Geometry: see drawing. Coordinates: mm, zero at the bounding-box minimum. A direction names the side the tool comes from. Give positions to 0.01 mm unless a question says otherwise; leave off trailing zeros. Loops run counter-clockwise (first coordinate to the right, second up) from the corner with the lowest first, then second, coordinate; pieces in that order, holes last. Notation, with made-up numbers: M 89,17 L 98,17 A22 ccw 98,54 Z; hole C -4.5,6 d2. An arc over 180 degrees is marked long. Put each result on its own line as item: value.
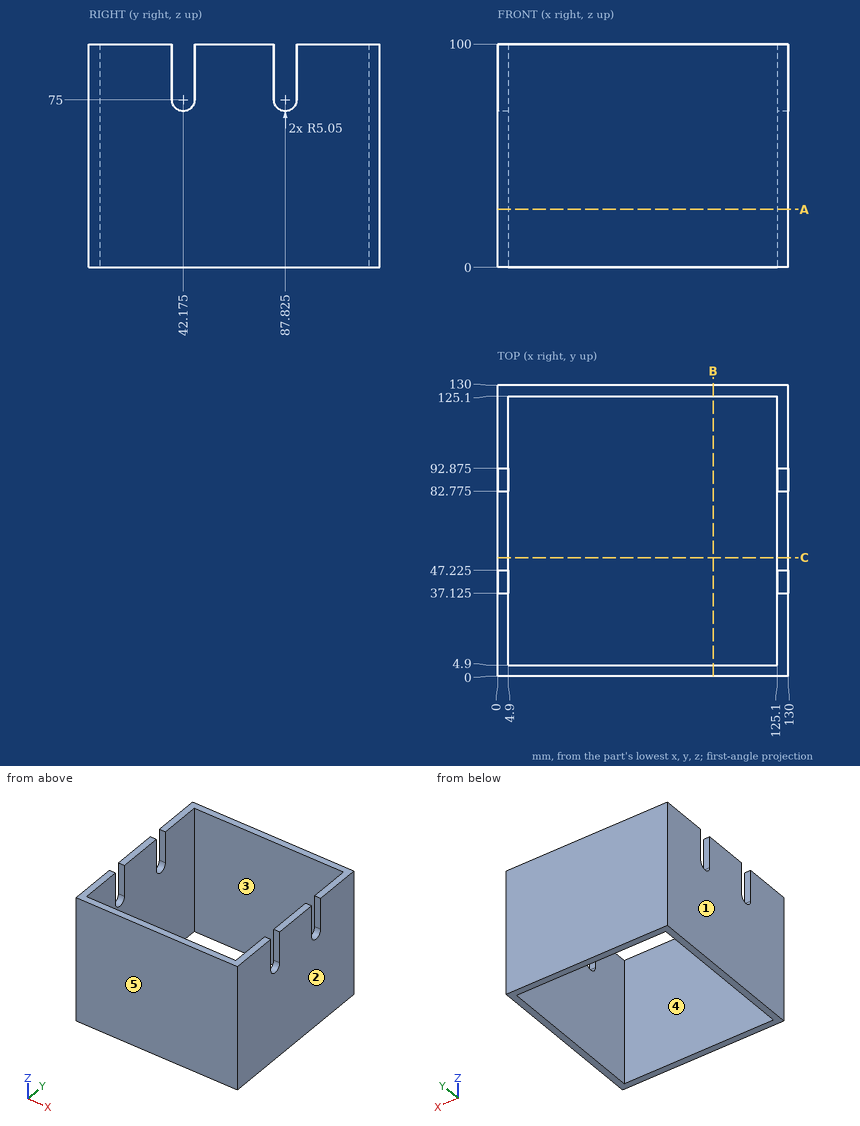
1. Section query A-A (z = 26). Output: boundary loops of the cut face in (x, y).
Found:
outline: M 0,0 L 130,0 L 130,130 L 0,130 Z; hole M 4.9,4.9 L 125.1,4.9 L 125.1,125.1 L 4.9,125.1 Z
2. Draft query along X for the marked faces 1, 2 and 3. Return one class per face: pulls with the +X half, pulls with the -X half, needs draft (parallel to the pull), parting line crosses it, or undercut.
Found:
face 1: pulls with the -X half
face 2: pulls with the +X half
face 3: undercut
3. Access query for the marked faces 4 and 5. Directions: +Z, -Z, +X, -X, +Y, -Y. A direction counts if a zero-diameter tool reaches every point of the face in a straight line with its end or side. Return the directions, or none.
Found:
face 4: +Z, -Z
face 5: +Z, -Z, +X, -X, -Y
4. Section query B-B (x = 96.5). Output: boundary loops of the cut face in (y, z).
Found:
outline: M 0,0 L 4.9,0 L 4.9,100 L 0,100 Z; M 125.1,0 L 130,0 L 130,100 L 125.1,100 Z
5. Material intervals for line 1 (X direction, y = 24.5, z = 90.5), sorted ascending. Write a range as from..to.
Found:
line 1: 0..4.9, 125.1..130
